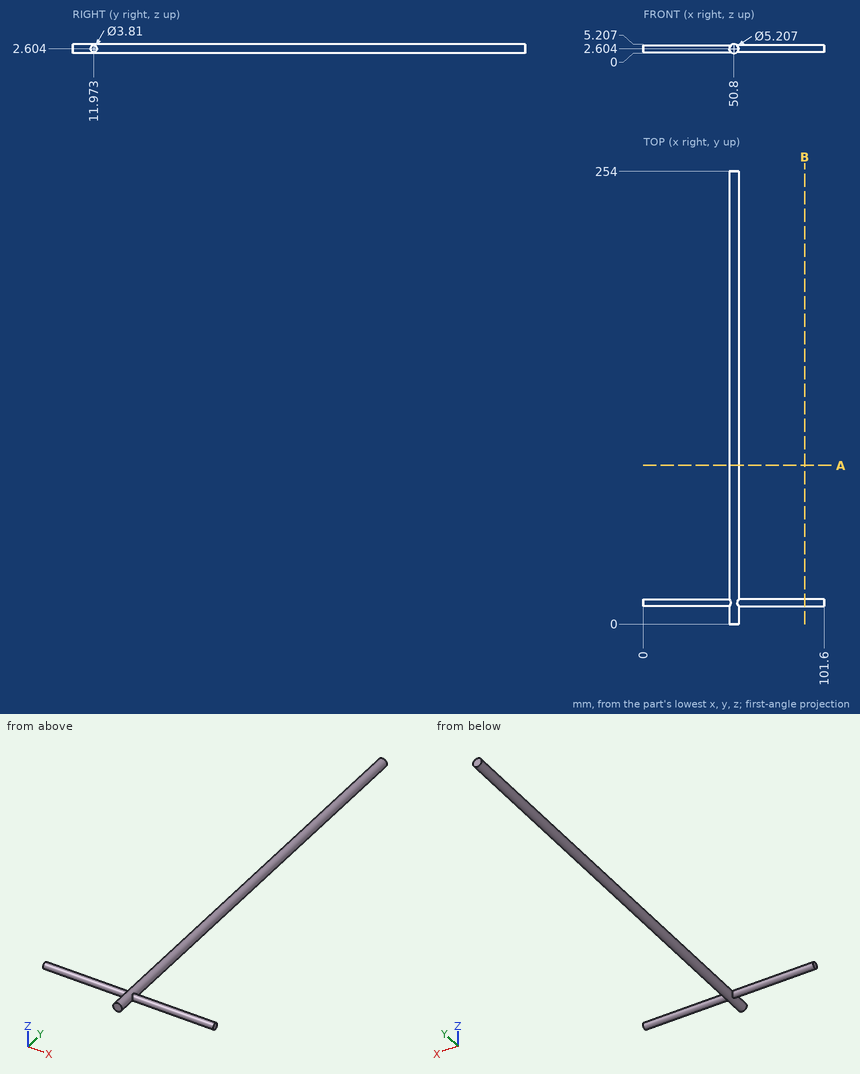
The drawing under review shows one solid part. Ordinate dimensions are in mm from its lowest x, y, z. Coordinates: 2 decimals unless noted, no trailing zeros. Order: outer loops, then holes, each group sorted by start corner. A loop starts at its lowest first (then second) coordinate and runs counter-clockwise, first axis right, second up. Notation, with made-up numbers: M 16.25,22 L 33.25,22 A11 ccw 33.25,33 Z; hole C 76,-27.75 d3. An arc over 180 degrees is marked long. Use a Markdown table: item, result.
(1) Add section A-A (y = 89). Give the boundary of the cut face in (x, z).
Worked answers:
| item | result |
|---|---|
| outline | C 50.8,2.6 d5.21 |
(2) For P1, Ø1, axis at x = 15.5, z = 4.5, coming from the +Y side; P2, Ø1, axis at y = 129, z = 0.5, coming from the +X side, all flat-tipped, find the tip position at first contact; note any pin that passes through.
Worked answers:
| item | result |
|---|---|
| P1 | stops at y = 13.27 |
| P2 | stops at x = 52.85 |
(3) Add section B-B (x = 90.5). Give the boundary of the cut face in (y, z) (1 decimal), then the cut area to 3 significant figures.
Worked answers:
| item | result |
|---|---|
| outline | C 12,2.6 d3.8 |
| area | 11.4 mm2 |
(4) Wall thickness on probe 1 along X at (y, z) = (71, 3); probe 2 along Y at (x, z) = (70.5, 2.3); probe 3 along X at (y, z) = (37.5, 4.5) (1 decimal): over which ranges is each line inside the solid? List them lowest first.
Worked answers:
| item | result |
|---|---|
| probe 1 | x = 48.23 to 53.37 |
| probe 2 | y = 10.09 to 13.85 |
| probe 3 | x = 49 to 52.6 |
